from build123d import *

# Parameters (mm, degrees)
F0_W         = 152.3266881704
F0_H         = 76.2925669551
F1_DEPTH     = 44.45
F2_T         = -2.54
F3_W         = 18.5941308737
F3_H         = 8.1849619746
F4_DEPTH     = 38.1
F5_T         = 2.54
F5_T3_DEPTH  = 13.2649619746
F5_T5_DEPTH  = 23.6741308737
F5_T7_DEPTH  = 78.8325669551
F5_T9_DEPTH  = 44.45
F5_T11_DEPTH = 152.3266881704
F7_R         = 5.6737308036
F8_DEPTH     = 89.211769402
F9_W         = 55.9205748141
F9_H         = 47.4143326283


# Not quite as in the source:
# - a shell that OpenCascade refuses in one call is made with other operations: the cavity is built on its own and cut out


with BuildPart() as f1:
    # F0 (on Front) → F1 (new body)
    with BuildSketch(Plane.XZ):
        with Locations((0.0222995877, 38.1462834775)):
            Rectangle(F0_W, F0_H)
    extrude(amount=F1_DEPTH)

    # F2
    f2_openings = [f1.faces().sort_by_distance(p)[0] for p in [
        (0.0223, -22.225, 0),
    ]]
    offset(amount=F2_T, openings=f2_openings)

    # F3 (on face) → F4 (join)
    with BuildSketch(Plane(origin=(-76.1410444975, 0, 0), x_dir=(0, -1, 0), z_dir=(-1, 0, 0))):
        with Locations((25.1720361412, 52.4518452585)):
            Rectangle(F3_W, F3_H)
    extrude(amount=F4_DEPTH)

    # F5: shell of thickness 2.54, made by hand


with BuildPart() as f5_core1:
    # F5_t2: copy of F1
    add(f1.part)

    # the walls: a layer under each face that stays
    f5_faces = [f5_core1.faces().sort_by_distance(p)[0] for p in [
        (0.0222995877, -22.225, 76.2925669551),
        (76.1856436729, -22.225, 38.1462834775),
        (-76.1410444975, -22.225, 38.1462834775),
        (0.0222995877, 0, 38.1462834775),
        (0.0222995877, -44.45, 38.1462834775),
        (-71.0634882251, -42.9683333333, 0),
        (-95.1910444975, -34.469101578, 52.4518452585),
        (-95.1910444975, -25.1720361412, 48.3593642712),
        (-95.1910444975, -15.8749707043, 52.4518452585),
        (-73.6010444975, -22.225, 36.8762834775),
        (0.0222995877, -2.54, 36.8762834775),
        (73.6456436729, -22.225, 36.8762834775),
        (0.0222995877, -41.91, 36.8762834775),
        (0.0222995877, -22.225, 73.7525669551),
    ]]
    thicken(f5_faces, amount=-F5_T, mode=Mode.SUBTRACT)

    # F5_s4 → F5_t3 (cut)
    with BuildSketch(Plane.XY.offset(45.8193642712)):
        Polygon((-76.1664444975, -34.494501578), (-73.6010444975, -34.469101578), (-73.6010444975, -31.929101578), (-76.1410444975, -31.929101578), align=None)
        Polygon((-76.1664444975, -15.8495707043), (-73.6010444975, -15.8749707043), (-73.6010444975, -18.4149707043), (-76.1410444975, -18.4149707043), align=None)
    extrude(amount=F5_T3_DEPTH, mode=Mode.SUBTRACT)

    # F5_s6 → F5_t5 (cut)
    with BuildSketch(Plane.XZ.offset(13.3349707043)):
        Polygon((-76.1664444975, 48.3339642712), (-73.6010444975, 48.3593642712), (-73.6010444975, 50.8993642712), (-76.1410444975, 50.8993642712), align=None)
    extrude(amount=F5_T5_DEPTH, mode=Mode.SUBTRACT)

    # F5_s8 → F5_t7 (cut)
    with BuildSketch(Plane.XY.offset(-2.54)):
        Polygon((-73.5756444975, -2.5654), (-76.1410444975, -2.54), (-76.1410444975, 0), (-73.6010444975, 0), align=None)
        Polygon((-73.5756444975, -41.8846), (-76.1410444975, -41.91), (-76.1410444975, -44.45), (-73.6010444975, -44.45), align=None)
        Polygon((73.6202436729, -2.5654), (73.6456436729, 0), (76.1856436729, 0), (76.1856436729, -2.54), align=None)
        Polygon((73.6202436729, -41.8846), (76.1856436729, -41.91), (76.1856436729, -44.45), (73.6456436729, -44.45), align=None)
    extrude(amount=F5_T7_DEPTH, mode=Mode.SUBTRACT)

    # F5_s10 → F5_t9 (cut)
    with BuildSketch(Plane.XZ):
        Polygon((-73.5756444975, 73.7271669551), (-76.1410444975, 73.7525669551), (-76.1410444975, 76.2925669551), (-73.6010444975, 76.2925669551), align=None)
        Polygon((73.6202436729, 73.7271669551), (76.1856436729, 73.7525669551), (76.1856436729, 76.2925669551), (73.6456436729, 76.2925669551), align=None)
    extrude(amount=F5_T9_DEPTH, mode=Mode.SUBTRACT)

    # F5_s12 → F5_t11 (cut)
    with BuildSketch(Plane.YZ.offset(-76.1410444975)):
        Polygon((-2.5654, 73.7271669551), (0, 73.7525669551), (0, 76.2925669551), (-2.54, 76.2925669551), align=None)
        Polygon((-41.8846, 73.7271669551), (-44.45, 73.7525669551), (-44.45, 76.2925669551), (-41.91, 76.2925669551), align=None)
    extrude(amount=F5_T11_DEPTH, mode=Mode.SUBTRACT)


with BuildPart() as f1_1:
    add(f1.part)

    # what is left inside the walls is the cavity
    f5_cavity = [f5_core1.part.solids().sort_by_distance(p)[0] for p in [
        (-101.541044, -25.172036, 56.518926),
    ]]
    add(f5_cavity, mode=Mode.SUBTRACT)


with BuildPart() as f8:
    # F7 (on Front) → F8 (new body)
    with BuildSketch(Plane.XZ):
        Circle(F7_R)
    extrude(amount=F8_DEPTH)

    # F9 (on Right) → F10 (revolve)
    with BuildSketch(Plane.YZ):
        with Locations((-43.1295465678, 23.7071663141)):
            Rectangle(F9_W, F9_H)
    revolve(axis=Axis((0, -43.1295465678, 0), (0, -1, 0)))


solid = f8.part
The model under review builds one solid part; all positions refer to its coordinate system, in mm. A direction names the side the tool comes from. Coordinates: 2 decimals unless noted, no trailing zeros. Loops run counter-clockwise (first coordinate to the right, second up) from the corner with the lowest first, then second, coordinate; pieces in that order, holes last.
(1) Consider section D-D, the plane y = -76.5. Give the boundary of the cut face in (x, z).
Determined:
outline: circle Ø11.35 at (0, 0)
(2) Tool access review of faces 1 (the flat face through (0, 0, 0)), 2 (the cylindrical face through (-4.182, -80.024, 3.835)), 3 (the cylindrical face through (-4.182, -7.478, 3.835)): name each direction out of +Z, -Z, +X, -X, +Y, -Y from which nothing blocks a thin tool from reaching the whole face with its end or side.
Determined:
face 1: +Z, -Z, +X, -X, +Y
face 2: -Y
face 3: +Y
(3) Consider section A-A, the plane x = 0. Give the boundary of the cut face in (y, z).
Determined:
outline: (-89.21, -5.67) - (-71.09, -5.67) - (-71.09, -47.41) - (-15.17, -47.41) - (-15.17, -5.67) - (0, -5.67) - (0, 5.67) - (-15.17, 5.67) - (-15.17, 47.41) - (-71.09, 47.41) - (-71.09, 5.67) - (-89.21, 5.67) - close
(4) Wall thickness on L1, parallel to Y at x = 7, z = -26; L2, parallel to Z at x = -22, y = -44.5; L3, parallel to X at y = -53, z = -20.5: over which ranges is each line inside the solid? List them lowest first.
Determined:
L1: y = -71.09 to -15.17
L2: z = -42 to 42
L3: x = -42.75 to 42.75
(5) Consider section C-C, the plane y = -40. Give the boundary of the cut face in (x, z), plus the area to 3 significant figures.
Determined:
outline: circle Ø94.83 at (0, 0)
area: 7,060 mm2
(6) Insertion check: P1, Ø10, axis at x = -21.5, y = -18, coming from the -Z side; P2, Ø4, axis at x = -4.5, y = -54, coming from the -Z side; P3, Ø10, axis at x = -37.5, y = -45, coming from the -Z side. Each pin has a flat end and moves straight along its axis. Give the tip position at first contact, or say it passes through.
Determined:
P1: stops at z = -44.45
P2: stops at z = -47.35
P3: stops at z = -34.52
(7) Consider section B-B, the plane z = 0. Give the boundary of the cut face in (x, y), plus the area to 3 significant figures.
Determined:
outline: (-47.41, -71.09) - (-5.67, -71.09) - (-5.67, -89.21) - (5.67, -89.21) - (5.67, -71.09) - (47.41, -71.09) - (47.41, -15.17) - (5.67, -15.17) - (5.67, 0) - (-5.67, 0) - (-5.67, -15.17) - (-47.41, -15.17) - close
area: 5,680 mm2
